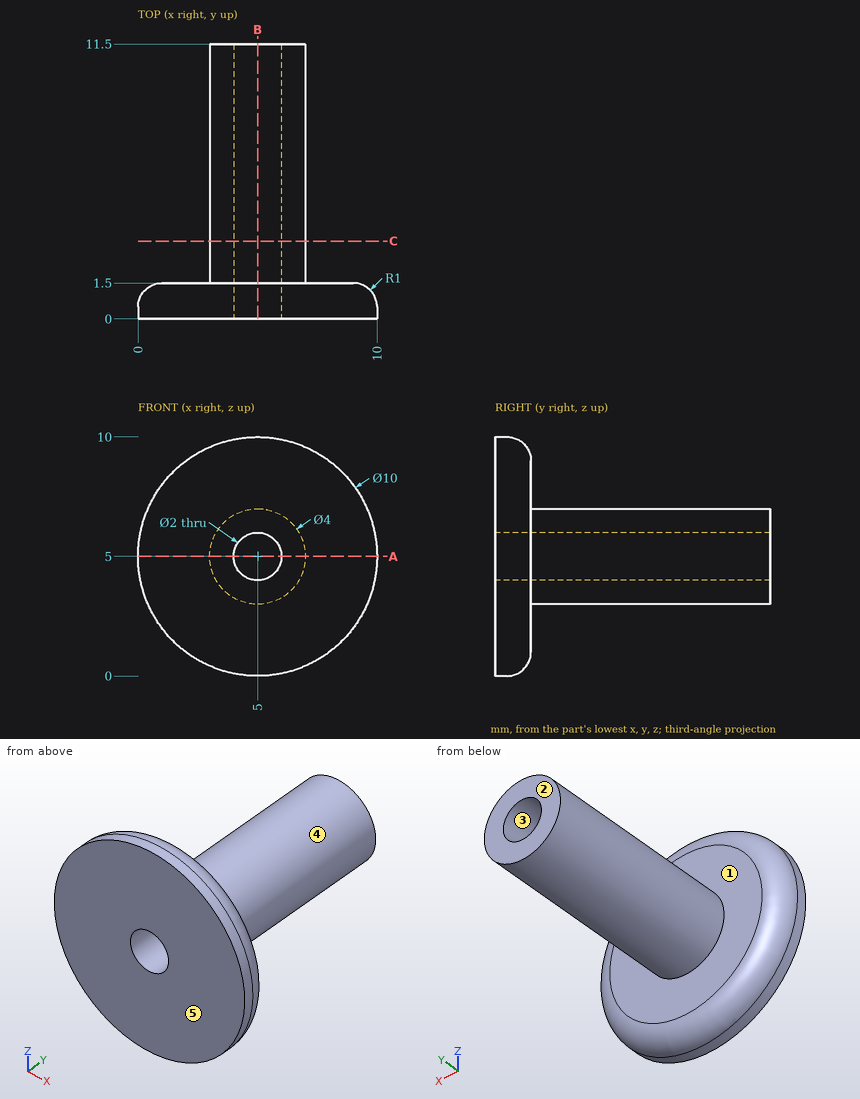
Answer from the drawing. Dimensions are ordinates in mm from the lowest x, y and z of the part. A direction names the side the tool comes from. Give positions to 0.01 mm unless a question says otherwise; leave off trailing zeros. Order: outer loops, then holes, each group sorted by start corner. A loop starts at its lowest first (then second) coordinate and runs counter-clockwise, first axis right, second up. Notation, with made-up numbers: (85, 4.5) -> (94, 4.5) arc R31 cw to (94, 35.5) -> close; hole circle Ø10 at (-33.5, 18). An arc over 180 degrees is marked (long way). One line per item, written item: value. Start each with the question number.
(1) For a pull along Z with two mould halves and no side action, classify the marked faces 3, 4 and 5 as released by +Z, released by -Z, zero draft, split by the parting line, or undercut.
(2) The part is cut by section A-A (z = 5). Determine the outline of the cut face in (x, y), and give its area (3 significant figures).
(3) Flat-ended cylindrical pins translate along their axes: P1, Ø1, axis at y = 8.5, z = 6.5, coming from the -X side; P2, Ø3, axis at y = 9, z = 6.5, coming from the +X side; P3, Ø3, axis at y = 4, z = 4.5, coming from the -X side. Find the tip coordinate at first contact, or state that the pin passes through.
(4) Straight lines are drawn through the part: L1, parallel to X at y = 3.5, z = 5; L2, parallel to Y at x = 6.25, z = 7.25; L3, parallel to Z at x = 6.5, y = 4. For each, find the intervals that lie inside material, in ascending order.
(5) A tool of negligible diameter and unlimited length cuts with its end or side. For the marked faces 1 and 2, from which of +Z, -Z, +X, -X, +Y, -Y can it reach the whole face along a straight path? Write none if from no direction.
(6) The part is cut by section B-B (x = 5). Determine the outline of the cut face in (y, z).
(7) The part is cut by section C-C (y = 3.25). Determine the outline of the cut face in (x, z).
Taken from the geometry:
1. face 3: undercut
1. face 4: split by the parting line
1. face 5: zero draft
2. outline: (0, 0) -> (4, 0) -> (4, 11.5) -> (3, 11.5) -> (3, 1.5) -> (1, 1.5) arc R1 ccw to (0, 0.5) -> close; (6, 0) -> (10, 0) -> (10, 0.5) arc R1 ccw to (9, 1.5) -> (7, 1.5) -> (7, 11.5) -> (6, 11.5) -> close
2. area: 31.6 mm^2
3. P1: x = 3.27
3. P2: x = 7
3. P3: x = 3
4. L1: 3 to 4, 6 to 7
4. L2: 0 to 1.5
4. L3: 3.68 to 6.32
5. face 1: +Y
5. face 2: +Z, -Z, +X, -X, +Y
6. outline: (0, 0) -> (0.5, 0) arc R1 ccw to (1.5, 1) -> (1.5, 3) -> (11.5, 3) -> (11.5, 4) -> (0, 4) -> close; (0, 6) -> (11.5, 6) -> (11.5, 7) -> (1.5, 7) -> (1.5, 9) arc R1 ccw to (0.5, 10) -> (0, 10) -> close
7. outline: circle Ø4 at (5, 5); hole circle Ø2 at (5, 5)
